Can you work these out from the drawing? Everything is in mm from the part's minimum corner. A direction names the side the tool comes from. Coordinates: 2 decimals unless noted, no trailing zeros. Loops run counter-clockwise (first coordinate to the right, second up) from the corner with the lowest first, then second, coordinate; pieces in that order, holes last.
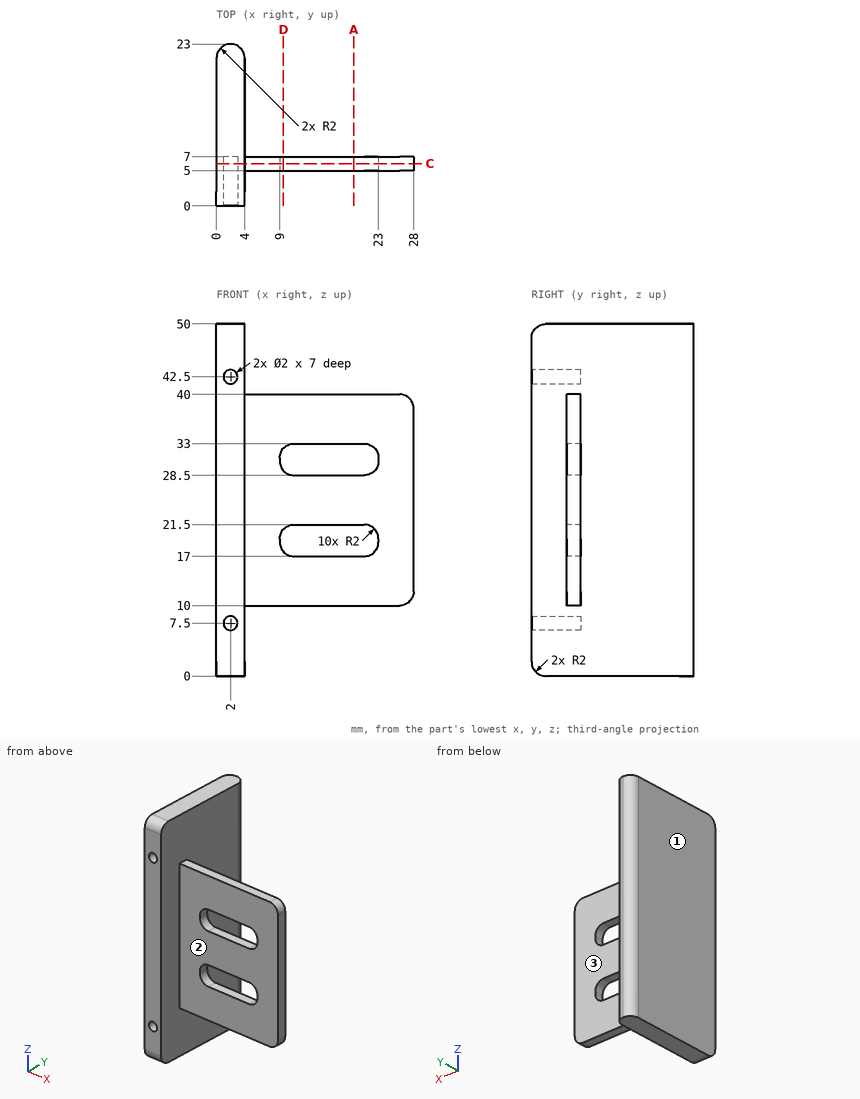
(1) Imagine slicing it at A-A, the plane x = 19.5. Write out the boundary of the cut face in (y, z), and give its area (3 significant figures).
Answers:
outline: (5, 10) - (7, 10) - (7, 17) - (5, 17) - close; (5, 21.5) - (7, 21.5) - (7, 28.5) - (5, 28.5) - close; (5, 33) - (7, 33) - (7, 40) - (5, 40) - close
area: 42.0 mm2
(2) Which directions (+Z, -Z, +X, -X, +Y, -Y) give clear straight access to the entire face, cutting with the end or side of a thin tool? Please do the marked faces 1, 2 and 3.
Answers:
face 1: +Z, -Z, -X, +Y, -Y
face 2: +Z, -Z, +X, -Y
face 3: +Z, -Z, +X, +Y
(3) Imagine slicing it at D-D, the plane x = 9.5. Write out the boundary of the cut face in (y, z), and give its area (3 significant figures).
Answers:
outline: (5, 10) - (7, 10) - (7, 17.68) - (5, 17.68) - close; (5, 20.82) - (7, 20.82) - (7, 29.18) - (5, 29.18) - close; (5, 32.32) - (7, 32.32) - (7, 40) - (5, 40) - close
area: 47.4 mm2
(4) Imagine slicing it at C-C, the plane y = 6. Write out the boundary of the cut face in (x, z), and give its area (3 significant figures).
Answers:
outline: (0, 0) - (4, 0) - (4, 10) - (26, 10) arc R2 ccw to (28, 12) - (28, 38) arc R2 ccw to (26, 40) - (4, 40) - (4, 50) - (0, 50) - close; hole circle Ø2 at (2, 7.5); hole circle Ø2 at (2, 42.5); hole (9, 19) arc R2 ccw to (11, 17) - (21, 17) arc R2 ccw to (23, 19) - (23, 19.5) arc R2 ccw to (21, 21.5) - (11, 21.5) arc R2 ccw to (9, 19.5) - close; hole (9, 30.5) arc R2 ccw to (11, 28.5) - (21, 28.5) arc R2 ccw to (23, 30.5) - (23, 31) arc R2 ccw to (21, 33) - (11, 33) arc R2 ccw to (9, 31) - close
area: 793 mm2
(5) I need wall thicknesses on probe 1 along Z at (x, y) = (11, 5.25); probe 2 along X at (y, z) = (5, 42.5); probe 3 along Y at (x, z) = (4.25, 36). Which ranges of each line are inside material? Lowest first, please.
Answers:
probe 1: z = 10 to 17, 21.5 to 28.5, 33 to 40
probe 2: x = 0 to 1, 3 to 4
probe 3: y = 5 to 7
(6) For pin 1 (12 mm diameter, centred on x = 12, z = 28, fed in from +Y); pin 2 (1 mm diameter, centred on x = 13.5, y = 6, fed in from +Z); pin 3 (2 mm diameter, centred on x = 18, y = 6, fed in from -Z); pin 4 (3 mm diameter, centred on x = 10.5, y = 2.5, fed in from +Z), each with a flat end and sliding along its axis, tell me the tip position at first contact or that it passes through.
Answers:
pin 1: stops at y = 7
pin 2: stops at z = 40
pin 3: stops at z = 10
pin 4: passes through
